```python
from build123d import *

# Parameters (mm, degrees)
BOSS_EXTRUDE1_DEPTH = 10
SKETCH5_R           = 1.4
CUT_EXTRUDE2_DEPTH  = 6
SKETCH4_R           = 1.75
CUT_EXTRUDE1_DEPTH  = 4.5
SKETCH6_R           = 1.75
SKETCH6_R_2         = 2.125
BOSS_EXTRUDE3_DEPTH = 5
BOSS_EXTRUDE4_START = -4
SKETCH6_3_R         = 1.75
BOSS_EXTRUDE4_DEPTH = 1
CUT_EXTRUDE3_DEPTH  = 5
SKETCH8_W           = 10
SKETCH8_H           = 11
CUT_EXTRUDE4_DEPTH  = 3
SKETCH10_R          = 1.4
BOSS_EXTRUDE5_DEPTH = 3
CHAMFER1_SIZE       = 2
FILLET1_R           = 1
CHAMFER2_SIZE       = 1.35
CHAMFER3_SIZE       = 6
SKETCH12_R          = 1.65
CUT_EXTRUDE6_DEPTH  = 61.634148794
CHAMFER4_SIZE       = 1.6


with BuildPart() as part:
    # Sketch2 → Boss-Extrude1 (new body)
    with BuildSketch(Plane.XY):
        Polygon((11.5, -6.2), (20, -6.2), (20, 9.8), (-20, 9.8), (-20, -6.2), (-11.5, -6.2), (-11.5, 6.2), (11.5, 6.2), align=None)
    extrude(amount=-BOSS_EXTRUDE1_DEPTH)

    # Sketch5 → Cut-Extrude2 (cut)
    with BuildSketch(Plane.XY):
        with Locations((15, -0.3)):
            Circle(SKETCH5_R)
    extrude(amount=-CUT_EXTRUDE2_DEPTH, mode=Mode.SUBTRACT)

    # Sketch4 → Cut-Extrude1 (cut)
    with BuildSketch(Plane.XZ.offset(6.2)):
        with Locations(Location((-17.25, -5, 0), (0, 0, 270))):
            Circle(SKETCH4_R)
        with Locations(Location((17.25, -5, 0), (0, 0, 270))):
            Circle(SKETCH4_R)
    extrude(amount=-CUT_EXTRUDE1_DEPTH, mode=Mode.SUBTRACT)

    # Sketch6 → Boss-Extrude3 (add)
    with BuildSketch(Plane.XZ.offset(6.2)):
        Polygon((-11.5, -10), (-20, -10), (-20, -26.5), (-9.5, -26.5), (-9.5, -54.5), (-2, -54.5), (20, -41.789296909), (20, -10), (11.5, -10), (11.5, -21.5), (-11.5, -21.5), align=None)
        with Locations(Location((-5.75, -28.5, 0), (0, 0, 270))):
            Circle(SKETCH6_R, mode=Mode.SUBTRACT)
        with Locations(Location((-5.75, -39.625, 0), (0, 0, 270))):
            Circle(SKETCH6_R_2, mode=Mode.SUBTRACT)
        with Locations(Location((-5.75, -50.75, 0), (0, 0, 270))):
            Circle(SKETCH6_R, mode=Mode.SUBTRACT)
        with Locations(Location((16.25, -39.625, 0), (0, 0, 270))):
            Circle(SKETCH6_R_2, mode=Mode.SUBTRACT)
    extrude(amount=-BOSS_EXTRUDE3_DEPTH)

    # Sketch6<3> → Boss-Extrude4 (add)
    with BuildSketch(Plane.XZ.offset(6.2).offset(BOSS_EXTRUDE4_START)):
        with Locations(Location((-5.75, -50.75, 0), (0, 0, 270))):
            Circle(SKETCH6_3_R)
        with Locations(Location((-5.75, -28.5, 0), (0, 0, 270))):
            Circle(SKETCH6_3_R)
    extrude(amount=-BOSS_EXTRUDE4_DEPTH)

    # Sketch7 → Cut-Extrude3 (cut)
    with BuildSketch(Plane(origin=(0, 0, -10), x_dir=(-1, 0, 0), z_dir=(0, 0, -1))):
        Polygon((11.5, -1.2), (11.5, -6.2), (15.5, -6.2), (20, -1.2), align=None)
    extrude(amount=CUT_EXTRUDE3_DEPTH, mode=Mode.SUBTRACT)

    # Sketch8 → Cut-Extrude4 (cut)
    with BuildSketch(Plane.ZY.offset(20)):
        with Locations((-5, 4.3)):
            Rectangle(SKETCH8_W, SKETCH8_H)
    extrude(amount=-CUT_EXTRUDE4_DEPTH, mode=Mode.SUBTRACT)

    # Sketch10 → Boss-Extrude5 (add)
    with BuildSketch(Plane.ZY.offset(17)):
        with BuildLine():
            Line((0, 6.2), (18.4, 6.2))
            Line((18.4, 6.2), (18.4, 23.7))
            Line((18.4, 23.7), (-10, 23.7))
            Line((-10, 23.7), (-10, -1.2))
            Line((-10, -1.2), (0, -1.2))
            Line((0, -1.2), (0, 3.320204103))
            ThreePointArc((0, 3.320204103), (-2.4, 4.3), (0, 5.279795897))
            Line((0, 5.279795897), (0, 6.2))
        make_face()
        with Locations(Location((-1, 20.3, 0), (0, 0, 270))):
            Circle(SKETCH10_R, mode=Mode.SUBTRACT)
        with Locations(Location((15, 20.3, 0), (0, 0, 270))):
            Circle(SKETCH10_R, mode=Mode.SUBTRACT)
    extrude(amount=-BOSS_EXTRUDE5_DEPTH)

    # Chamfer1
    chamfer1_edges = [part.edges().sort_by_distance(p)[0] for p in [
        (-15.5, 6.2, 18.4),
        (-15.5, 23.7, -10),
        (-15.5, 23.7, 18.4),
    ]]
    chamfer(chamfer1_edges, length=CHAMFER1_SIZE)

    # Fillet1
    fillet1_edges = [part.edges().sort_by_distance(p)[0] for p in [
        (-11.5, -3.7, -15),
        (20, 1.8, 0),
        (-20, -3.7, 0),
        (11.5, 0, 0),
        (-17, 2.5, 0),
        (-11.5, 0, -10),
        (20, 4.3, -10),
        (-9.5, -3.7, -54.5),
        (-9.5, -3.7, -26.5),
        (-20, -3.7, -26.5),
        (20, -3.7, -41.789296909),
        (11.5, 2.5, -10),
        (-11.5, 0, 0),
    ]]
    fillet(fillet1_edges, radius=FILLET1_R)

    # Chamfer2
    chamfer2_edges = [part.edges().sort_by_distance(p)[0] for p in [
        (-5.75, -6.2, -37.5),
        (16.25, -6.2, -37.5),
    ]]
    chamfer(chamfer2_edges, length=CHAMFER2_SIZE)

    # Chamfer3
    chamfer3_edges = [part.edges().sort_by_distance(p)[0] for p in [
        (-14, 9.8, -5),
    ]]
    chamfer(chamfer3_edges, length=CHAMFER3_SIZE)

    # Sketch12 → Cut-Extrude6 (cut, through all)
    with BuildSketch(Plane.XZ.offset(-6.2)):
        with Locations(Location((0, -5, 0), (0, 0, 270))):
            Circle(SKETCH12_R)
    extrude(amount=-CUT_EXTRUDE6_DEPTH, mode=Mode.SUBTRACT)

    # Chamfer4
    chamfer4_edges = [part.edges().sort_by_distance(p)[0] for p in [
        (0, 6.2, -3.35),
    ]]
    chamfer(chamfer4_edges, length=CHAMFER4_SIZE)


solid = part.part
```
Here's how the part is built. I have some questions about the finished solid (model axes, mm). A direction names the side the tool comes from. Round coordinates to 2 decimals unless told otherwise and drop trailing zeros. Order: outer loops, then holes, each group sorted by start corner. A loop starts at its lowest first (then second) coordinate and runs counter-clockwise, first axis right, second up. Notation, with made-up numbers: M 14.25,-11 L 31.25,-11 A28 ccw 31.25,7 Z; hole C 64.25,77 d9. An arc over 180 degrees is marked long. One line per question, with ' | ' between items.
1) For pin 1 Ø4 at (y, z) = (11, 7.5) entering from +X; pin 2 Ø1 at (x, y) = (13.5, 12) entering from -Z; pin 3 Ø5.5 at (y, z) = (-4.5, -37.5) entering from -X; pin 4 Ø0.8 at (x, y) = (15, -0.5) entering from +Z, each with a flat end and sliding along its axis, tell me the tip position at first contact or that it passes through.
Working result:
pin 1: x = -14 | pin 2: through | pin 3: x = -9.5 | pin 4: z = -6
2) I want a section at A-A, the plane y = -0.3. Write out the boundary of the cut face in (x, z).
Working result:
outline: M -17,-10 L -12.5,-10 A1 ccw -11.5,-9 L -11.5,-1 A1 ccw -12.5,0 L -16,0 A1 ccw -17,-1 Z; M 11.5,-9 A1 ccw 12.5,-10 L 19,-10 A1 ccw 20,-9 L 20,-1 A1 ccw 19,0 L 16.4,0 L 16.4,-6 L 13.6,-6 L 13.6,0 L 12.5,0 A1 ccw 11.5,-1 Z
3) I want a section at D-D, the plane z = -28.5. Write out the boundary of the cut face in (x, y).
Working result:
outline: M -9.5,-6.2 L -7.5,-6.2 L -7.5,-2.2 L -4,-2.2 L -4,-6.2 L 20,-6.2 L 20,-1.2 L -9.5,-1.2 Z
4) I want a section at B-B, the plane x = -5.75. Write out the boundary of the cut face in (y, z).
Working result:
outline: M -6.2,-54.5 L -1.2,-54.5 L -1.2,-41.75 L -4.85,-41.75 L -6.2,-43.1 L -6.2,-49 L -2.2,-49 L -2.2,-52.5 L -6.2,-52.5 Z; M -6.2,-36.15 L -4.85,-37.5 L -1.2,-37.5 L -1.2,-21.5 L -6.2,-21.5 L -6.2,-26.75 L -2.2,-26.75 L -2.2,-30.25 L -6.2,-30.25 Z; M 6.2,-10 L 9.8,-10 L 9.8,0 L 6.2,0 Z
5) I want a section at C-C, the plane y = 11.5. Write out the boundary of the cut face in (x, z), then the cut area to 3 significant figures.
Working result:
outline: M -17,-10 L -9.7,-10 L -9.7,0 L -14,0 L -14,18.4 L -17,18.4 Z | area: 128 mm²
6) If we mould it in two halves opening along X, with no side actions, what happens to faces 1 (the face through (-15.5, 22.7, 17.4)), 2 (the face through (-6, -2.2, -28))? For each: +X half, -X half, draft (parallel to the pull), parting line (faces both ways), or undercut.
Working result:
face 1: draft | face 2: undercut
7) I need wall thicknesses on line 1 along Z through (x, y) = (-16.2, 20.3); line 2 along X through (y, z) = (-2.75, -40.5); line 3 along Z through (x, y) = (-13.5, 6.75). Which ranges of each line are inside material? Lowest first, please.
Working result:
line 1: -10 to -2.4, 0.4 to 13.6, 16.4 to 18.4 | line 2: -9.5 to -7.69, -3.81 to 14.31, 18.19 to 20 | line 3: -10 to 0
8) For faces 3 (the face through (11.5, -1.5, -8.8)), 4 (the face through (15, 0, -6)), 5 (the face through (-15.52, 21.33, 15.95)), 6 (the face through (-17, -1.7, -5)), which set-ups out of +Z, -Z, +X, -X, +Y, -Y let a thin tool reach every point of the face, with its end or its side?
Working result:
face 3: +Z, -Y | face 4: +Z | face 5: +X, -X | face 6: -Y
